Check sheet for the modelled part. Datum: model origin and axes. Units: mm. Coordinates: 2 decimals unless noted, no trailing zeros. Write each loop counter-clockwise with the first axis right and the second up, starting at its lowest first coordinate (ties: lowest second). Pieces come first, ordered by that corner, then holes. Notation, with made-up numbers: (13, 52) - (64, 52) arc R32 cw to (64, 85) - close; hole circle Ø8 at (21.25, 67). An arc over 180 degrees is marked (long way). Use one line per item in the form item = value. Start each with the question number.
1. Cross-section at B-B on y = 2.5. Record the boundary of the cut face in (x, z).
2. Go/stop test with flat-tipped pins: pin 1 Ø1 at (x, y) = (-19, 1) entering from +Z; pin 2 Ø1 at (x, y) = (-21.5, 4) entering from -Z. Record where each tip stops, or that it passes through.
3. Cross-section at A-A on x = -20. Record the boundary of the cut face in (y, z), then the cut area to 3 significant figures.
4. Scan lines: line 1 along Z through (x, y) = (-21.55, 1.55); line 2 along Y through (x, z) = (-20, -38); line 3 along Z through (x, y) = (-21.55, 2.6). Record each from-to range of solid material in increasing order.
5. Draft check along Z on faces 1 (the face through (-21.5, 2.57, -24.65)), 2 (the face through (-20, 3, 1.5)), 3 (the face through (-20, 3, -51.5)). Enter one of: +Z half, -Z half, draft (parallel to the pull), parting line (faces both ways), or undercut.
6. Cross-section at C-C on z = -8.5. Record the boundary of the cut face in (x, y), then the cut area to 3 significant figures.
```python
from build123d import *

# Parameters (mm, degrees)
ESBO_O1_R                = 1.5
RESSALTO_EXTRUS_O1_DEPTH = 50
ESBO_O2_R                = 2
RESSALTO_EXTRUS_O2_DEPTH = 1.5
RESSALTO_EXTRUS_O3_START = -51.5
ESBO_O2_2_R              = 2
RESSALTO_EXTRUS_O3_DEPTH = 1.5
FILETE1_R                = 0.7


with BuildPart() as part:
    # Esboço1 → Ressalto-extrusão1 (new body)
    with BuildSketch(Plane.XY):
        with Locations((-20, 2.5)):
            Circle(ESBO_O1_R)
    extrude(amount=-RESSALTO_EXTRUS_O1_DEPTH)

    # Esboço2 → Ressalto-extrusão2 (add)
    with BuildSketch(Plane.XY):
        with Locations((-20, 2.5)):
            Circle(ESBO_O2_R)
    extrude(amount=RESSALTO_EXTRUS_O2_DEPTH)

    # Esboço2<2> → Ressalto-extrusão3 (add)
    with BuildSketch(Plane.XY.offset(RESSALTO_EXTRUS_O3_START)):
        with Locations((-20, 2.5)):
            Circle(ESBO_O2_2_R)
    extrude(amount=RESSALTO_EXTRUS_O3_DEPTH)

    # Filete1
    # the kernel refuses this fillet: 0.7 mm, written as the material it takes off along each edge
    with BuildSketch(Plane(origin=(-20, 2.5, 0), x_dir=(1, 0, 0), z_dir=(0, -1, 0))) as filete1_piece_1:
        with BuildLine():
            CenterArc((1.3, 0.670820393), FILETE1_R, 286.601549599, 73.398450401)
            Line((2, 0.670820393), (2.014, 0.670820393))
            Line((2.014, 0.670820393), (2.014, 0))
            Line((2.014, 0), (2, -0.014))
            ThreePointArc((2, -0.014), (1.75, -0.014), (1.504, -0.013416408))
            Line((1.504, -0.013416408), (1.5, 0))
        make_face()
    revolve(axis=Axis((-20, 2.5, 0), (0, 0, 1)), mode=Mode.SUBTRACT)
    with BuildSketch(Plane(origin=(-20, 2.5, 1.5), x_dir=(1, 0, 0), z_dir=(0, -1, 0))) as filete1_piece_2:
        with BuildLine():
            CenterArc((2 - FILETE1_R, -FILETE1_R), FILETE1_R, 0, 90)
            Line((2 - FILETE1_R, 0), (2 - FILETE1_R, FILETE1_R * 0.02))
            Line((2 - FILETE1_R, FILETE1_R * 0.02), (2 + FILETE1_R * 0.02, FILETE1_R * 0.02))
            Line((2 + FILETE1_R * 0.02, FILETE1_R * 0.02), (2 + FILETE1_R * 0.02, -FILETE1_R))
            Line((2 + FILETE1_R * 0.02, -FILETE1_R), (2, -FILETE1_R))
        make_face()
    revolve(axis=Axis((-20, 2.5, 1.5), (0, 0, 1)), mode=Mode.SUBTRACT)
    with BuildSketch(Plane(origin=(-20, 2.5, -50), x_dir=(1, 0, 0), z_dir=(0, -1, 0))) as filete1_piece_3:
        with BuildLine():
            CenterArc((1.3, -0.670820393), FILETE1_R, 0, 73.398450401)
            Line((1.5, 0), (1.504, 0.013416408))
            ThreePointArc((1.504, 0.013416408), (1.75, 0.014), (2, 0.014))
            Line((2, 0.014), (2.014, 0))
            Line((2.014, 0), (2.014, -0.670820393))
            Line((2.014, -0.670820393), (2, -0.670820393))
        make_face()
    revolve(axis=Axis((-20, 2.5, -50), (0, 0, 1)), mode=Mode.SUBTRACT)
    with BuildSketch(Plane(origin=(-20, 2.5, -51.5), x_dir=(1, 0, 0), z_dir=(0, -1, 0))) as filete1_piece_4:
        with BuildLine():
            CenterArc((2 - FILETE1_R, FILETE1_R), FILETE1_R, 270, 90)
            Line((2 - FILETE1_R, 0), (2 - FILETE1_R, -FILETE1_R * 0.02))
            Line((2 - FILETE1_R, -FILETE1_R * 0.02), (2 + FILETE1_R * 0.02, -FILETE1_R * 0.02))
            Line((2 + FILETE1_R * 0.02, -FILETE1_R * 0.02), (2 + FILETE1_R * 0.02, FILETE1_R))
            Line((2 + FILETE1_R * 0.02, FILETE1_R), (2, FILETE1_R))
        make_face()
    revolve(axis=Axis((-20, 2.5, -51.5), (0, 0, 1)), mode=Mode.SUBTRACT)


solid = part.part
```
Final values:
q1.outline = (-22, -50.8) arc R0.7 ccw to (-21.3, -51.5) - (-18.7, -51.5) arc R0.7 ccw to (-18, -50.8) - (-18, -50.67) arc R0.7 ccw to (-18.5, -50) - (-18.5, 0) arc R0.7 ccw to (-18, 0.67) - (-18, 0.8) arc R0.7 ccw to (-18.7, 1.5) - (-21.3, 1.5) arc R0.7 ccw to (-22, 0.8) - (-22, 0.67) arc R0.7 ccw to (-21.5, 0) - (-21.5, -50) arc R0.7 ccw to (-22, -50.67) - close
q2.pin_1 = 1.5
q2.pin_2 = -51.42
q3.outline = (0.5, -50.8) arc R0.7 ccw to (1.2, -51.5) - (3.8, -51.5) arc R0.7 ccw to (4.5, -50.8) - (4.5, -50.67) arc R0.7 ccw to (4, -50) - (4, 0) arc R0.7 ccw to (4.5, 0.67) - (4.5, 0.8) arc R0.7 ccw to (3.8, 1.5) - (1.2, 1.5) arc R0.7 ccw to (0.5, 0.8) - (0.5, 0.67) arc R0.7 ccw to (1, 0) - (1, -50) arc R0.7 ccw to (0.5, -50.67) - close
q3.area = 161 mm²
q4.line_1 = -51.27 to -50.2, 0.2 to 1.27
q4.line_2 = 1 to 4
q4.line_3 = -51.45 to -50.02, 0.02 to 1.45
q5.face_1 = undercut
q5.face_2 = +Z half
q5.face_3 = -Z half
q6.outline = circle Ø3 at (-20, 2.5)
q6.area = 7.07 mm²
